Job drawing, mm, ordinate dimensions from the low corner. One solid piece. Give positions to 0.01 mm unless a question says otherwise; leave off trailing zeros. Loops run counter-clockwise (first coordinate to the right, second up) from the corner with the lowest first, then second, coordinate; pieces in that order, holes last. Notation, with made-up numbers: (84, 17) - (123, 17) arc R21 cw to (123, 31) - close; hole circle Ø7 at (49.25, 72.25). An arc over 180 degrees is marked (long way). Answer as CSV lines item,"result". Start each with the question number.
Item 1: Saw through at D-D on x = 62.8. Give the cut face in (y, z), plus the area to 3 significant figures.
Item 2: Drill centre lines: L1, parallel to X at y = 53.5, z = 1.35; L2, parallel to Y at x = 62.8, z = 0.8; L3, parallel to Y at x = 3, z = 0.9. Where is each one in solid material? Low to high. Write a range as from..to.
Item 3: Saw through at C-C on x = 44. Give the cut face in (y, z), plus the area to 3 significant figures.
Item 4: Saw through at A-A on y = 54.6. Give the cut face in (x, z), plus the area to 3 significant figures.
Item 5: Pin check, flat tip, straight feed: pin 1 (2.5 mm diameter, centred on x = 79, y = 60.6, fed in from +Z). Stop position of the tip, or through.
Item 6: Saw through at B-B on z = 0.4. State how many separate pieces and enclosed holes the cut face has, plus the area to 3 significant figures.
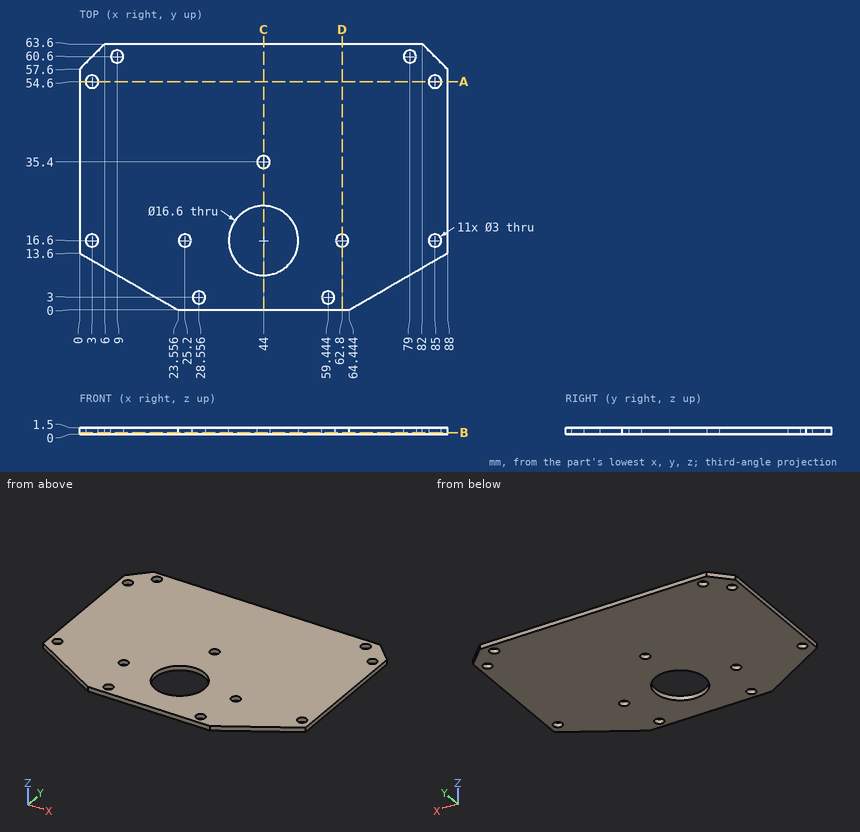
Responses:
1,outline,"(0, 0) - (15.1, 0) - (15.1, 1.5) - (0, 1.5) - close; (18.1, 0) - (63.6, 0) - (63.6, 1.5) - (18.1, 1.5) - close"
1,area,"90.9 mm2"
2,L1,"0..1.98, 4.02..83.98, 86.02..88"
2,L2,"0..15.1, 18.1..63.6"
2,L3,"11.87..15.1, 18.1..53.1, 56.1..60.6"
3,outline,"(0, 0) - (8.3, 0) - (8.3, 1.5) - (0, 1.5) - close; (24.9, 0) - (33.9, 0) - (33.9, 1.5) - (24.9, 1.5) - close; (36.9, 0) - (63.6, 0) - (63.6, 1.5) - (36.9, 1.5) - close"
3,area,"66.0 mm2"
4,outline,"(0, 0) - (1.5, 0) - (1.5, 1.5) - (0, 1.5) - close; (4.5, 0) - (83.5, 0) - (83.5, 1.5) - (4.5, 1.5) - close; (86.5, 0) - (88, 0) - (88, 1.5) - (86.5, 1.5) - close"
4,area,"123 mm2"
5,pin 1,"through"
6,separate pieces,"1"
6,enclosed holes,"12"
6,area,"4,950 mm2"
